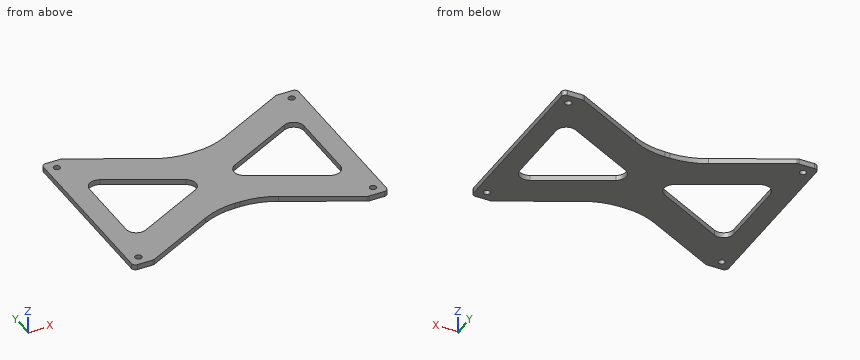
```python
from build123d import *

# Parameters (mm, degrees)
SKETCH1_R           = 2.032
BOSS_EXTRUDE1_DEPTH = 3.302
FILLET1_R           = 45.72
FILLET2_R           = 2.54
CUT_EXTRUDE1_DEPTH  = 106.174191833
FILLET3_R           = 6.35


with BuildPart() as part:
    # Sketch1 → Boss-Extrude1 (new body)
    with BuildSketch(Plane.XY):
        Polygon((-79.375, 68.922542022), (-79.375, -41.313457978), (-66.675, -41.313457978), (-12.7, -13.38067482), (12.7, -13.38067482), (66.675, -41.313457978), (79.375, -41.313457978), (79.375, 68.922542022), (66.675, 68.922542022), (12.7, 40.989758863), (-12.7, 40.989758863), (-66.675, 68.922542022), align=None)
        with Locations(Location((-73.025, 62.572542022, 0), (0, 0, 180))):
            Circle(SKETCH1_R, mode=Mode.SUBTRACT)
        with Locations(Location((-73.025, -34.963457978, 0), (0, 0, 180))):
            Circle(SKETCH1_R, mode=Mode.SUBTRACT)
        with Locations(Location((73.025, -34.963457978, 0), (0, 0, 180))):
            Circle(SKETCH1_R, mode=Mode.SUBTRACT)
        with Locations(Location((73.025, 62.572542022, 0), (0, 0, 180))):
            Circle(SKETCH1_R, mode=Mode.SUBTRACT)
    extrude(amount=BOSS_EXTRUDE1_DEPTH)

    # Fillet1
    fillet1_edges = [part.edges().sort_by_distance(p)[0] for p in [
        (-12.7, 40.989758863, 1.651),
        (12.7, 40.989758863, 1.651),
        (12.7, -13.38067482, 1.651),
        (-12.7, -13.38067482, 1.651),
    ]]
    fillet(fillet1_edges, radius=FILLET1_R)

    # Fillet2
    fillet2_edges = [part.edges().sort_by_distance(p)[0] for p in [
        (-66.675, 68.922542022, 1.651),
        (66.675, 68.922542022, 1.651),
        (79.375, 68.922542022, 1.651),
        (79.375, -41.313457978, 1.651),
        (66.675, -41.313457978, 1.651),
        (-66.675, -41.313457978, 1.651),
        (-79.375, -41.313457978, 1.651),
        (-79.375, 68.922542022, 1.651),
    ]]
    fillet(fillet2_edges, radius=FILLET2_R)

    # Sketch2 → Cut-Extrude1 (cut, through all)
    with BuildSketch(Plane.XY.offset(3.302)):
        Polygon((-66.675, 46.062542022), (-66.675, -18.453457978), (-4.342308693, 13.804542022), align=None)
        Polygon((66.675, 46.062542022), (66.675, -18.453457978), (4.342308693, 13.804542022), align=None)
    extrude(amount=-CUT_EXTRUDE1_DEPTH, mode=Mode.SUBTRACT)

    # Fillet3
    fillet3_edges = [part.edges().sort_by_distance(p)[0] for p in [
        (-4.342308693, 13.804542022, 1.651),
        (-66.675, -18.453457978, 1.651),
        (-66.675, 46.062542022, 1.651),
        (4.342308693, 13.804542022, 1.651),
        (66.675, 46.062542022, 1.651),
        (66.675, -18.453457978, 1.651),
    ]]
    fillet(fillet3_edges, radius=FILLET3_R)


solid = part.part
```
The listing builds one solid part. Answer for the finished solid, in the listing's coordinates (mm). Give positions to 0.01 mm unless a question says otherwise; leave off trailing zeros. Order: outer loops, then holes, each group sorted by start corner. A loop starts at its lowest first (then second) coordinate and runs counter-clockwise, first axis right, second up. Notation, with made-up numbers: (31, 27.5) -> (85, 27.5) arc R21 cw to (85, 42.5) -> close; hole circle Ø6 at (-24, 17.25). An arc over 180 degrees is marked (long way). One line per item, written item: value.
1) Flat-ended cylindrical pins translate along their axes: P1, Ø0.9, axis at x = -0.5, z = 1.5, coming from the +Y side; P2, Ø1, axis at x = -32.5, z = 2, coming from the +Y side; P3, Ø0.9, axis at x = 0, z = 2, coming from the -Y side. Find the tip coordinate at first contact, or state that the pin passes through.
Reported:
P1: stops at y = 40.99
P2: stops at y = 51.5
P3: stops at y = -13.38
2) Find the intervals of material crossed by line 1 (X direction, y = 18, z = 2.1) (3 decimals); line 2 (X direction, y = 61, z = 1.85) (3 decimals); line 3 (X direction, y = -2.5, z = 2.4) (3 decimals), in increasing order.
Reported:
line 1: x = -79.375 to -66.675, -13.392 to 13.392, 66.675 to 79.375
line 2: x = -79.375 to -74.312, -71.738 to -51.366, 51.366 to 71.738, 74.312 to 79.375
line 3: x = -79.375 to -66.675, -35.848 to 35.848, 66.675 to 79.375
3) Find section D-D, the plane y = 0. Determine the outline of the cut face in (x, z) (3 decimals), plus the area to 3 significant figures.
Reported:
outline: (-79.375, 0) -> (-66.675, 0) -> (-66.675, 3.302) -> (-79.375, 3.302) -> close; (-31.017, 0) -> (31.017, 0) -> (31.017, 3.302) -> (-31.017, 3.302) -> close; (66.675, 0) -> (79.375, 0) -> (79.375, 3.302) -> (66.675, 3.302) -> close
area: 289 mm^2
4) Find section B-B, the plane x = -34.5. Determine the outline of the cut face in (y, z), plus the area to 3 significant figures.
Reported:
outline: (-24.66, 0) -> (-1.8, 0) -> (-1.8, 3.3) -> (-24.66, 3.3) -> close; (29.41, 0) -> (52.27, 0) -> (52.27, 3.3) -> (29.41, 3.3) -> close
area: 151 mm^2
5) Find section C-C, the plane y = 58.5. Determine the outline of the cut face in (x, z) (3 decimals), plus the area to 3 significant figures.
Reported:
outline: (-79.375, 0) -> (-46.535, 0) -> (-46.535, 3.302) -> (-79.375, 3.302) -> close; (46.535, 0) -> (79.375, 0) -> (79.375, 3.302) -> (46.535, 3.302) -> close
area: 217 mm^2
6) Find section A-A, the plane y = 21.5. Determine the outline of the cut face in (x, z) (3 decimals).
Reported:
outline: (-79.375, 0) -> (-66.675, 0) -> (-66.675, 3.302) -> (-79.375, 3.302) -> close; (-19.212, 0) -> (19.212, 0) -> (19.212, 3.302) -> (-19.212, 3.302) -> close; (66.675, 0) -> (79.375, 0) -> (79.375, 3.302) -> (66.675, 3.302) -> close
